Verification items for the finished model (mm, model axes). A direction names the side the tool comes from. Round coordinates to 2 decimals unless told otherwise and drop trailing zeros. Order: outer loops, then holes, each group sorted by start corner. A loop starts at its lowest first (then second) coordinate and runs counter-clockwise, first axis right, second up. Notation, with made-up numbers: (83.25, 16.5) -> (123.25, 16.5) arc R24 cw to (123.25, 47.5) -> close; hole circle Ø11 at (81.25, 50.25). An arc over 180 degrees is marked (long way). Return JSON: item names as keys, results as strings. Group by question number.
Item 1: Access from +Z, -Z, +X, -X, +Y, -Y to the whole of each face (thin tool, end or side, straight path). Record for faces 1 (the flat face through (-31, 5, -5.5)), 2 (the cylindrical face through (-4.88, -0.25, -1.08)), 3 (the flat face through (-4, 10.5, -2)).
Item 2: Sectioned sample at D-D on y = 1. Give the number of separate pieces and of enclosed holes in the cut face, plus the area to 3 significant figures.
Item 3: Depth check by flat-ended pin: pin 1 Ø6.5 at (x, z) = (-3, -3.5) entering from +Y; pin 2 Ø7 at (x, y) = (-8.5, 5) entering from -Z; pin 3 Ø8 at (x, y) = (-7, 9) entering from +Z; pin 4 Ø5 at (x, z) = (9.5, -5.5) entering from -Y. Enter the tip coordinate at first touch or a pass-through.
Item 4: Sectioned sample at B-B on y = 12.75. Record the cut outline in (x, z), plus the area to 3 significant figures.
Item 5: Scan lines: probe 1 along X at (y, z) = (4.5, -5); probe 2 along Y at (x, z) = (-22.5, 1); probe 3 along X at (y, z) = (3.75, -4.75). Record each from-to range of solid material in increasing order. Write a range as from..to.
Item 6: Sectioned sample at A-A on x = 0. Record the cut outline in (y, z).
Item 7: Sectioned sample at C-C on z = -11.25. Record the cut outline in (x, y), plus the area to 3 significant figures.
```python
from build123d import *

# Parameters (mm, degrees)
SKETCH_1_R      = 2.525
SKETCH_1_R_2    = 2.505
EXTRUDE_1_DEPTH = 10
SKETCH_2_R      = 1.525
EXTRUDE_2_DEPTH = 5
SKETCH_5_R      = 3.99
EXTRUDE_4_DEPTH = 9
FILLET_1_R      = 4
FILLET_2_R      = 2
FILLET_3_R      = 2
SKETCH_6_R      = 5
EXTRUDE_5_DEPTH = 0.5


with BuildPart() as part:
    # 草图1 → 凸台-拉伸1 (new body)
    with BuildSketch(Plane(origin=(0, 0, 0), x_dir=(1, 0, 0), z_dir=(0, 1, 0))):
        with BuildLine():
            Line((-5.123475383, -4), (-28.225082782, -4))
            ThreePointArc((-28.225082782, -4), (-37.111262075, -2.031009601), (-32, 5.5))
            Line((-32, 5.5), (-28, 5.5))
            Line((-28, 5.5), (-28, 16.482886319))
            Line((-28, 16.482886319), (-13.123475383, 4))
            Line((-13.123475383, 4), (-5.123475383, 4))
            ThreePointArc((-5.123475383, 4), (6.5, 0), (-5.123475383, -4))
        make_face()
        with Locations(Location((-32, 0, 0), (0, 0, 270))):
            Circle(SKETCH_1_R, mode=Mode.SUBTRACT)
        with Locations(Location((-23.339745962, 5, 0), (0, 0, 270))):
            Circle(SKETCH_1_R_2, mode=Mode.SUBTRACT)
    extrude(amount=EXTRUDE_1_DEPTH)

    # 草图2 → 凸台-拉伸2 (add, symmetric)
    with BuildSketch(Plane(origin=(0, 5, 0), x_dir=(1, 0, 0), z_dir=(0, 1, 0))):
        with BuildLine():
            ThreePointArc((4.159420521, -4.994919512), (6.496753335, -0.205416905), (4.466659496, 4.722176717))
            add(Edge.make_bspline(
                [(4.466659496, 4.722176717), (7.284864094, 2.056465312), (15.716737601, -2.396247552), (20.490071148, 0)],
                knots=[0, 0, 0, 0, 1, 1, 1, 1], degree=3))
            ThreePointArc((20.490071148, 0), (24.593372298, -1.499185377), (22.849655998, -5.50469291))
            add(Edge.make_bspline(
                [(4.159420521, -4.994919512), (15.25095487, -8.232572742), (22.849655998, -5.50469291)],
                knots=[0, 0, 0, 1, 1, 1], degree=2))
        make_face()
        with Locations(Location((21.836015336, -2.681125555, 0), (0, 0, 90))):
            Circle(SKETCH_2_R, mode=Mode.SUBTRACT)
    extrude(amount=EXTRUDE_2_DEPTH, both=True)

    # 草图5 → 凸台-拉伸4 (add, symmetric)
    with BuildSketch(Plane(origin=(0, 5, 0), x_dir=(1, 0, 0), z_dir=(0, 1, 0))):
        with Locations(Location((0, 0, 0), (0, 0, 270))):
            Circle(SKETCH_5_R)
    extrude(amount=EXTRUDE_4_DEPTH, both=True)

    # 圆角1
    fillet_1_edges = [part.edges().sort_by_distance(p)[0] for p in [
        (-13.123475383, 5, -4),
    ]]
    fillet(fillet_1_edges, radius=FILLET_1_R)

    # 圆角2
    fillet_2_edges = [part.edges().sort_by_distance(p)[0] for p in [
        (-28, 5, -16.482886319),
    ]]
    fillet(fillet_2_edges, radius=FILLET_2_R)

    # 圆角3
    fillet_3_edges = [part.edges().sort_by_distance(p)[0] for p in [
        (-28, 5, -5.5),
    ]]
    fillet(fillet_3_edges, radius=FILLET_3_R)

    # 草图6 → 凸台-拉伸5 (add)
    with BuildSketch(Plane(origin=(0, 10, 0), x_dir=(1, 0, 0), z_dir=(0, 1, 0))):
        with Locations(Location((0, 0, 0), (0, 0, 270))):
            Circle(SKETCH_6_R)
    extrude_5 = extrude(amount=EXTRUDE_5_DEPTH)

    # 镜向1: 凸台-拉伸5 across plane
    add(extrude_5.mirror(Plane.ZX.offset(5)))


solid = part.part
```
Recorded:
{
 "1": {"face 1": "-Z, -X, +Y, -Y", "face 2": "-Y", "face 3": "+Y"},
 "2": {"separate pieces": "1", "enclosed holes": "3", "area": "565 mm²"},
 "3": {"pin 1": "y = 14", "pin 2": "z = -4.15", "pin 3": "z = 5.77", "pin 4": "through"},
 "4": {"outline": "circle Ø7.98 at (0, 0)", "area": "50.0 mm²"},
 "5": {"probe 1": "-34.29..-25.84, -20.83..-14.32, -4.15..4.15", "probe 2": "0..10", "probe 3": "-34.77..-25.83, -20.85..-14, -4.44..4.44"},
 "6": {"outline": "(-4, -3.99) -> (-0.5, -3.99) -> (-0.5, -5) -> (0, -5) -> (0, -6.5) -> (10, -6.5) -> (10, -5) -> (10.5, -5) -> (10.5, -3.99) -> (14, -3.99) -> (14, 3.99) -> (10.5, 3.99) -> (10.5, 5) -> (10, 5) -> (10, 6.5) -> (0, 6.5) -> (0, 5) -> (-0.5, 5) -> (-0.5, 3.99) -> (-4, 3.99) -> close"},
 "7": {"outline": "(-28, 0) -> (-21.76, 0) -> (-21.76, 10) -> (-28, 10) -> close", "area": "62.4 mm²"}
}
